from build123d import *

# Parameters (mm, degrees)
SKETCH1_W           = 9.57
SKETCH1_H           = 2.25
SKETCH1_W_2         = 5.5
SKETCH1_H_2         = 0.35
BOSS_EXTRUDE1_DEPTH = 0.24
FILLET1_R           = 1


with BuildPart() as part:
    # Sketch1 → Boss-Extrude1 (new body)
    with BuildSketch(Plane(origin=(0, 0, 0), x_dir=(1, 0, 0), z_dir=(0, 1, 0))):
        with Locations((4.785, 1.125)):
            Rectangle(SKETCH1_W, SKETCH1_H)
        with Locations((3.27, 1.575)):
            Rectangle(SKETCH1_W_2, SKETCH1_H_2, mode=Mode.SUBTRACT)
        with Locations((6.57, 0.275)):
            Rectangle(SKETCH1_W_2, SKETCH1_H_2, mode=Mode.SUBTRACT)
    extrude(amount=BOSS_EXTRUDE1_DEPTH)

    # Fillet1
    fillet1_edges = [part.edges().sort_by_distance(p)[0] for p in [
        (0, 0.12, -2.25),
        (9.57, 0.12, -2.25),
    ]]
    fillet(fillet1_edges, radius=FILLET1_R)


solid = part.part
Can you work these out from the model? Positions are in its coordinate system, mm. Coordinates: 2 decimals unless noted, no trailing zeros. Loops run counter-clockwise (first coordinate to the right, second up) from the corner with the lowest first, then second, coordinate; pieces in that order, holes last. Notation, with made-up numbers: M 32,9 L 89,9 A31 ccw 89,33 Z; hole C -35,-5 d9. An arc over 180 degrees is marked long. Return JSON: item names as keys, results as strings. Group by question number.
Item 1: Imagine slicing it at A-A (z = -0.3). Please give me the cut outline in (x, y).
Item 2: Imagine slicing it at D-D (x = 7.5). Please give me the cut outline in (y, z), and give its area (3 significant figures).
Item 3: If I drill on L1, parallel to Z at x = 1, y = 0.1; L2, parallel to X at y = 0.2, z = -0.15; L3, parallel to X at y = 0.15, z = -1.7, over which ranges is the centre line in solid material (lowest first)? Write a range as from..to.
Item 4: Imagine slicing it at C-C (x = 4.25). Please give me the cut outline in (y, z), and give its area (3 significant figures).
Item 5: Imagine slicing it at B-B (y = 0.1). Please give me the cut outline in (x, z).
Verdict:
{
 "1": {"outline": "M 0,0 L 3.82,0 L 3.82,0.24 L 0,0.24 Z; M 9.32,0 L 9.57,0 L 9.57,0.24 L 9.32,0.24 Z"},
 "2": {"outline": "M 0,-2.25 L 0.24,-2.25 L 0.24,-0.45 L 0,-0.45 Z; M 0,-0.1 L 0.24,-0.1 L 0.24,0 L 0,0 Z", "area": "0.456 mm^2"},
 "3": {"L1": "z = -2.25..-1.75, -1.4..0", "L2": "x = 0..3.82, 9.32..9.57", "L3": "x = 0.11..0.52, 6.02..9.46"},
 "4": {"outline": "M 0,-2.25 L 0.24,-2.25 L 0.24,-1.75 L 0,-1.75 Z; M 0,-1.4 L 0.24,-1.4 L 0.24,-0.45 L 0,-0.45 Z; M 0,-0.1 L 0.24,-0.1 L 0.24,0 L 0,0 Z", "area": "0.372 mm^2"},
 "5": {"outline": "M 0,-1.25 A1 ccw 1,-2.25 L 8.57,-2.25 A1 ccw 9.57,-1.25 L 9.57,0 L 0,0 Z; hole M 0.52,-1.75 L 6.02,-1.75 L 6.02,-1.4 L 0.52,-1.4 Z; hole M 3.82,-0.45 L 9.32,-0.45 L 9.32,-0.1 L 3.82,-0.1 Z"}
}
